Here's the drawing with two shaded views (mm, measured from the low corner). I have some questions. A direction names the side the tool comes from. Round coordinates to 2 decimals unless told otherwise and drop trailing zeros. Loops run counter-clockwise (first coordinate to the right, second up) from the corner with the lowest first, then second, coordinate; pieces in that order, holes last.
(1) I want a section at C-C on y = 8.75. Write out the boundary of the cut face in (x, z).
(2) Will these pins go through, and if not, where does the flat tip stop? pin 1 Ø2 at (x, z) = (4.5, 3) entering from -Y; pin 2 Ø2 at (y, z) = (4, 1) entering from +X; pin 3 Ø2 at (y, z) = (3, 1) entering from +X.
(3) I want a section at D-D on x = 13. Write out the boundary of the cut face in (y, z) (1 decimal).
(4) I want a section at B-B on z = 3.3. Write out the boundary of the cut face in (x, y).
(5) I want a section at A-A on x = 10.25. Write out the boundary of the cut face in (y, z).
(6) If I drill on line 1 along X through (y, z) = (8, 1) (1 decimal); line 2 along X through (y, z) = (14.5, 1.95) (1 decimal); line 3 along Z through (x, y) = (12.5, 13.5), over which ranges is the centre line in solid material (lowest first)?
(7) Which directions (+Z, -Z, +X, -X, +Y, -Y) give clear straight access to the entire face, cutting with the end or side of a thin tool? Please do the marked faces 1, 2 and 3.
(8) Thinking about a two-plate mould opening in X: for the marked faces 4, 5 and 6, which applies, released by +X, released by -X, zero draft, split by the parting line, or undercut?
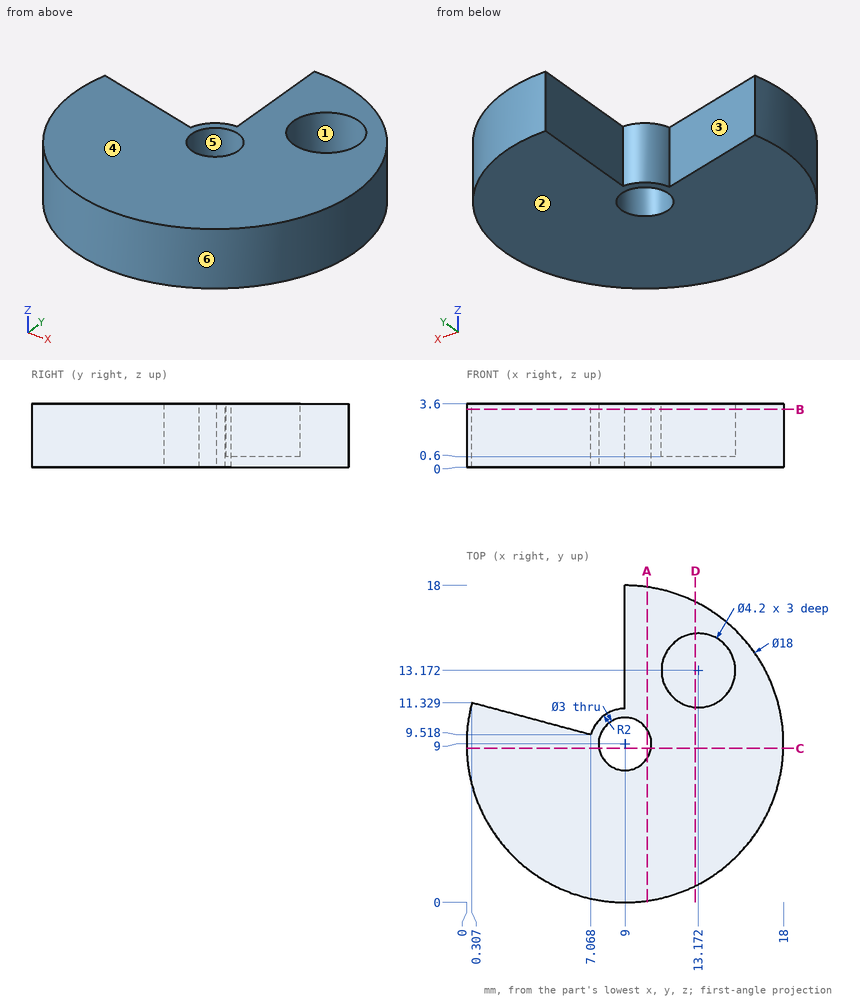
Filled sheet:
1. outline: (0, 0) - (7.52, 0) - (7.52, 3.6) - (0, 3.6) - close; (10.48, 0) - (18, 0) - (18, 3.6) - (10.48, 3.6) - close
2. pin 1: stops at y = 0.71
2. pin 2: stops at x = 17.06
2. pin 3: stops at x = 16.48
3. outline: (0.9, 0) - (17.1, 0) - (17.1, 3.6) - (15.3, 3.6) - (15.3, 0.6) - (11.1, 0.6) - (11.1, 3.6) - (0.9, 3.6) - close
4. outline: (0.31, 11.33) arc R9 ccw (long way) to (9, 18) - (9, 11) arc R2 ccw to (7.07, 9.52) - close; hole circle Ø3 at (9, 9); hole circle Ø4.2 at (13.17, 13.17)
5. outline: (0.09, 0) - (8.17, 0) - (8.17, 3.6) - (0.09, 3.6) - close; (9.83, 0) - (17.91, 0) - (17.91, 3.6) - (9.83, 3.6) - close
6. line 1: x = 0.1 to 7.9, 10.1 to 17.9
6. line 2: x = 9 to 11.5, 14.8 to 16.1
6. line 3: z = 0 to 0.6
7. face 1: +Z
7. face 2: -Z, +X, -X, +Y, -Y
7. face 3: +Z, -Z, +Y
8. face 4: zero draft
8. face 5: undercut
8. face 6: split by the parting line
